Design review of the part shown in the three views and the two pictorial views. Dimensions are in mm from the part's minimum x, y and z. A direction names the side the tool comes from. Coordinates: 2 decimals unless noted, no trailing zeros. Order: outer loops, then holes, each group sorted by start corner. A loop starts at its lowest first (then second) coordinate and runs counter-clockwise, first axis right, second up. Notation, with made-up numbers: (35.25, 82.5) -> (71.25, 82.5) arc R19 cw to (71.25, 117.5) -> close; hole circle Ø11 at (44.5, -34.5). An arc over 180 degrees is marked (long way). Answer as a JSON object with one key per item and string values. Group by question number.
1) Machinability: for the marked faces 1 and 2, which of the approach directions +Z, -Z, +X, -X, +Y, -Y give a long, thin tool a straight path to every point of the face, cutting with its end or side? Answer none if there is none.
2) Add section A-A, the plane x = 8. Write out the cut boundary in (y, z), then the cut area to 3 significant figures.
3) Add section B-B, the plane z = 5. Write out the cut boundary in (x, y).
4) Add section C-C, the plane y = 7.25. Write out the cut boundary in (x, z).
5) For pin 1 (4 mm diameter, centred on x = 8, z = 5, fed in from -Y); pin 2 (5 mm diameter, centred on x = 8.5, y = 7.5, fed in from +Z); pin 3 (1 mm diameter, centred on x = 7.5, z = 27, fed in from -Y); pin 4 (3 mm diameter, centred on x = 6.5, z = 6, fed in from +Y), all flat-tipped, find the tip position at first contact; note any pin that passes through.
6) Add section D-D, the plane z = 34.5. Write out the cut boundary in (x, y), then the cut area to 3 significant figures.
7) Draft analysis for pull direction Y (two halves, no side actions). For the marked faces 3, 4 and 5, state which applies: +Y half, -Y half, draft (parallel to the pull), parting line (faces both ways), or undercut.
8) Wall thickness on L1, parallel to Z at x = 8, y = 6.15; L2, parallel to Y at x = 8, z = 66; L3, parallel to Z at x = 8, y = 3.2: over which ranges is each line inside the solid? List them lowest first.
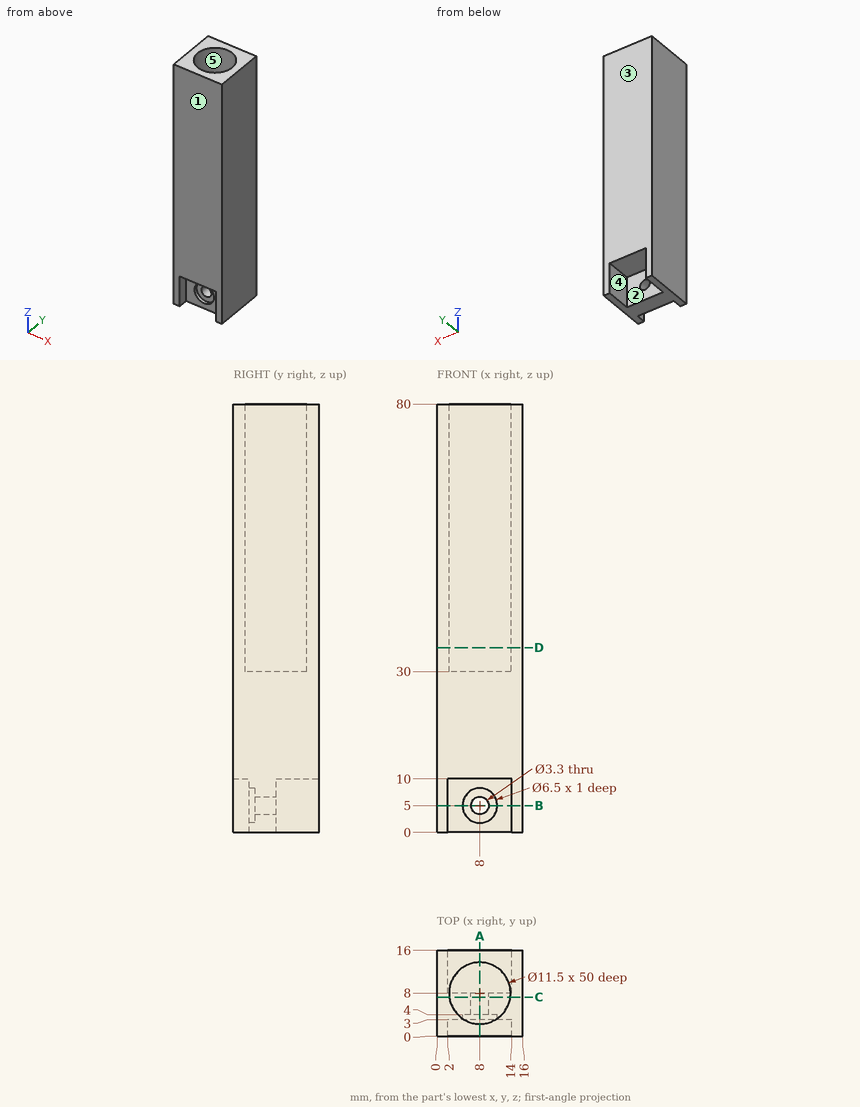
Output values:
{
 "1": {"face 1": "+Z, -Z, +X, -X, -Y", "face 2": "-Z, +Y"},
 "2": {"outline": "(0, 10) -> (3, 10) -> (3, 8.25) -> (4, 8.25) -> (4, 6.65) -> (8, 6.65) -> (8, 10) -> (16, 10) -> (16, 80) -> (13.75, 80) -> (13.75, 30) -> (2.25, 30) -> (2.25, 80) -> (0, 80) -> close; (3, 0) -> (8, 0) -> (8, 3.35) -> (4, 3.35) -> (4, 1.75) -> (3, 1.75) -> close", "area": "575 mm²"},
 "3": {"outline": "(0, 0) -> (2, 0) -> (2, 3) -> (4.75, 3) -> (4.75, 4) -> (6.35, 4) -> (6.35, 8) -> (2, 8) -> (2, 16) -> (0, 16) -> close; (9.65, 4) -> (11.25, 4) -> (11.25, 3) -> (14, 3) -> (14, 0) -> (16, 0) -> (16, 16) -> (14, 16) -> (14, 8) -> (9.65, 8) -> close"},
 "4": {"outline": "(0, 0) -> (16, 0) -> (16, 80) -> (13.7, 80) -> (13.7, 30) -> (2.3, 30) -> (2.3, 80) -> (0, 80) -> close; hole circle Ø3.3 at (8, 5)"},
 "5": {"pin 1": "stops at y = 4", "pin 2": "stops at z = 30", "pin 3": "stops at y = 0", "pin 4": "stops at y = 8"},
 "6": {"outline": "(0, 0) -> (16, 0) -> (16, 16) -> (0, 16) -> close; hole circle Ø11.5 at (8, 8)", "area": "152 mm²"},
 "7": {"face 3": "+Y half", "face 4": "draft", "face 5": "undercut"},
 "8": {"L1": "z = 0 to 3.35, 6.65 to 30", "L2": "y = 0 to 2.25, 13.75 to 16", "L3": "z = 0 to 1.75, 8.25 to 30"}
}
